For this review, take the finished solid that the model builds, in its own axes (mm). Face numbers are marked on the shaded views. A direction names the side the tool comes from. Round coordinates to 2 decimals unless told otherwise and drop trailing zeros. Order: outer loops, then holes, each group sorted by start corner. A loop starts at its lowest first (then second) coordinate and runs counter-clockwise, first axis right, second up. Notation, with made-up numbers: (17, -33) -> (57, -33) arc R16 cw to (57, -28) -> close; hole circle Ø1 at (62, 39). An arc over 180 degrees is marked (long way). Use a Markdown table: item, result. Add a question column.
1) Wall thickness on line 1 along X through (y, z) = (-15.75, 16.75); line 2 along Z through (x, y) = (-24.7, -12.7) (3 decimals): over which ranges is each line inside the solid? List them lowest first. Write a range as [from, to].
2) Consider section C-C (y = -12.7). State the section outline as (x, z) points (3 decimals), plus the area to 3 significant figures.
3) Draft analysis for pull direction X (two halves, no side actions). For the marked faces 3, 4 and 5, state which applies: pulls with the +X half, pulls with the -X half, needs draft (parallel to the pull), parting line crosses it, or undercut.
4) Clearance check with flat-ended pins moving along their axes: P1, Ø3, axis at y = -12.5, z = 11.5, coming from the -X side; P2, Ø1, axis at x = -8, y = -17.5, coming from the +Z side; P3, Ø3, axis at y = -13, z = 13, coming from the +X side. State where each tip first meets the part, or that it passes through.
5) Consider section B-B (z = 12.7). State the section outline as (x, y) points (3 decimals), plus the area to 3 significant figures.
6) Machinability: for the marked faces 1 and 2, which of the approach directions +Z, -Z, +X, -X, +Y, -Y give a long, thin tool a straight path to every point of the face, cutting with its end or side? Answer none if there is none.
7) Consider section D-D (z = 23.5). State the section outline as (x, y) points.
8) Consider section A-A (x = -12.7). State the section outline as (y, z) points.
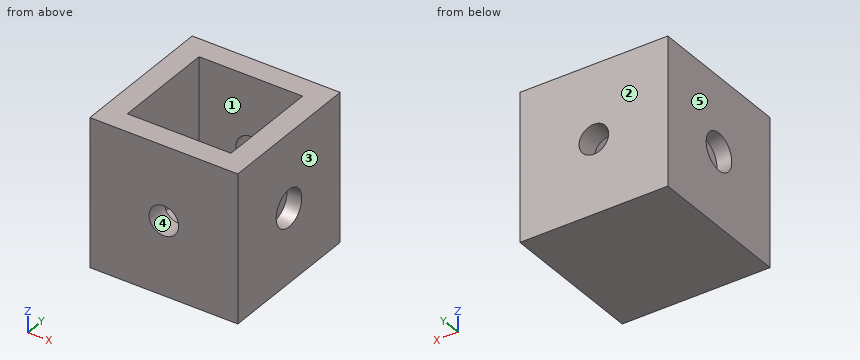
```python
from build123d import *

# Parameters (mm, degrees)
F0_W     = 25.4
F0_H     = 25.4
F1_DEPTH = 25.4
F2_T     = -3.81
F5_D     = 5.08
F5_DEPTH = 50.8
F4_R     = 3.175
F6_DEPTH = 2.54
F7_R     = 3.175
F8_DEPTH = 2.54


with BuildPart() as f1:
    # F0 (on Front) → F1 (new body)
    with BuildSketch(Plane.XZ):
        with Locations((-12.7, 12.7)):
            Rectangle(F0_W, F0_H)
    extrude(amount=F1_DEPTH)

    # F2
    f2_openings = [f1.faces().sort_by_distance(p)[0] for p in [
        (-12.7, -12.7, 25.4),
    ]]
    offset(amount=F2_T, openings=f2_openings)

    # F5
    with Locations(Plane.XZ.offset(25.4)):
        with Locations((-12.7, 12.7)):
            Hole(F5_D / 2, depth=F5_DEPTH)

    # F4 (on face) → F6 (cut)
    with BuildSketch(Plane.YZ):
        with Locations((-12.7, 12.7)):
            Circle(F4_R)
    extrude(amount=-F6_DEPTH, mode=Mode.SUBTRACT)

    # F7 (on face) → F8 (cut)
    with BuildSketch(Plane(origin=(-25.4, 0, 0), x_dir=(0, -1, 0), z_dir=(-1, 0, 0))):
        with Locations((12.7, 12.7)):
            Circle(F7_R)
    extrude(amount=-F8_DEPTH, mode=Mode.SUBTRACT)


solid = f1.part
```
Results list:
| question | item | result |
|---|---|---|
| 1 | line 1 | [-25.4, -21.59], [-3.81, 0] |
| 1 | line 2 | [0, 9.525], [15.875, 25.4] |
| 2 | outline | (-25.4, 0) -> (0, 0) -> (0, 9.525) -> (-2.54, 9.525) -> (-2.54, 15.875) -> (0, 15.875) -> (0, 25.4) -> (-3.81, 25.4) -> (-3.81, 3.81) -> (-21.59, 3.81) -> (-21.59, 25.4) -> (-25.4, 25.4) -> (-25.4, 15.875) -> (-22.86, 15.875) -> (-22.86, 9.525) -> (-25.4, 9.525) -> close |
| 2 | area | 229 mm2 |
| 3 | face 3 | pulls with the +X half |
| 3 | face 4 | undercut |
| 3 | face 5 | pulls with the -X half |
| 4 | P1 | x = -22.86 |
| 4 | P2 | z = 3.81 |
| 4 | P3 | x = -2.54 |
| 5 | outline | (-25.4, -25.4) -> (-15.24, -25.4) -> (-15.24, -21.59) -> (-21.59, -21.59) -> (-21.59, -3.81) -> (-15.24, -3.81) -> (-15.24, 0) -> (-25.4, 0) -> (-25.4, -9.525) -> (-22.86, -9.525) -> (-22.86, -15.875) -> (-25.4, -15.875) -> close; (-10.16, -25.4) -> (0, -25.4) -> (0, -15.875) -> (-2.54, -15.875) -> (-2.54, -9.525) -> (0, -9.525) -> (0, 0) -> (-10.16, 0) -> (-10.16, -3.81) -> (-3.81, -3.81) -> (-3.81, -21.59) -> (-10.16, -21.59) -> close |
| 5 | area | 258 mm2 |
| 6 | face 1 | +Z |
| 6 | face 2 | +Z, -Z, +X, -X, +Y |
| 7 | outline | (-25.4, -25.4) -> (0, -25.4) -> (0, 0) -> (-25.4, 0) -> close; hole (-21.59, -21.59) -> (-3.81, -21.59) -> (-3.81, -3.81) -> (-21.59, -3.81) -> close |
| 8 | outline | (-25.4, 0) -> (0, 0) -> (0, 10.16) -> (-3.81, 10.16) -> (-3.81, 3.81) -> (-21.59, 3.81) -> (-21.59, 10.16) -> (-25.4, 10.16) -> close; (-25.4, 15.24) -> (-21.59, 15.24) -> (-21.59, 25.4) -> (-25.4, 25.4) -> close; (-3.81, 15.24) -> (0, 15.24) -> (0, 25.4) -> (-3.81, 25.4) -> close |
